from build123d import *

# Parameters (mm, degrees)
F0_W      = 140
F0_H      = 180
F1_DEPTH  = 70
F2_W      = 130
F2_H      = 170
F3_DEPTH  = 65
F4_SIZE   = 45
F5_W      = 30
F5_H      = 49.6265143156
F6_DEPTH  = 25
F7_R      = 14.99999
F9_DEPTH  = 7
F10_W     = 59.1894394159
F10_H     = 26.9657306075
F11_DEPTH = 25
F12_W     = 90
F12_H     = 7
F13_DEPTH = 20
F14_W     = 90
F14_H     = 7
F15_DEPTH = 20
F17_DEPTH = 25
F19_DEPTH = 25
F20_R     = 5


# Not quite as in the source:
# - a fillet or chamfer is up to 0.001 mm smaller than in the source, because OpenCascade refuses the exact size


with BuildPart() as f1:
    # F0 (on Top) → F1 (new body)
    with BuildSketch(Plane.XY):
        with Locations((46.5964969993, 53.7995101511)):
            Rectangle(F0_W, F0_H)
    extrude(amount=F1_DEPTH)

    # F2 (on face) → F3 (cut)
    with BuildSketch(Plane(origin=(0, 0, 0), x_dir=(1, 0, 0), z_dir=(0, 0, -1))):
        with Locations((46.5964969993, -53.7995101511)):
            Rectangle(F2_W, F2_H)
    extrude(amount=-F3_DEPTH, mode=Mode.SUBTRACT)

    # F4
    f4_edges = [f1.edges().sort_by_distance(p)[0] for p in [
        (46.596497, 143.79951, 70),
        (46.596497, 138.79951, 65),
    ]]
    chamfer(f4_edges, length=F4_SIZE)

    # F5 (on face) → F6 (cut)
    with BuildSketch(Plane.XZ.offset(36.2004898489)):
        with Locations((46.5964969993, 24.8132571578)):
            Rectangle(F5_W, F5_H)
    extrude(amount=-F6_DEPTH, mode=Mode.SUBTRACT)

    # F7 (radius 15 in the source; OpenCascade refuses exactly that, so slightly less here)
    f7_edges = [f1.edges().sort_by_distance(p)[0] for p in [
        (61.596497, -33.70049, 49.626514),
        (31.596497, -33.70049, 49.626514),
    ]]
    fillet(f7_edges, radius=F7_R)

    # F8 (on face) → F9 (join)
    with BuildSketch(Plane(origin=(0, 0, 0), x_dir=(1, 0, 0), z_dir=(0, 0, -1))):
        Polygon((-23.4035030007, -28.7995101511), (-23.4035030007, -143.7995101511), (116.5964969993, -143.7995101511), (116.5964969993, -28.7995101511), (111.5964969993, -28.7995101511), (111.5964969993, -138.7995101511), (-18.4035030007, -138.7995101511), (-18.4035030007, -28.7995101511), align=None)
    extrude(amount=F9_DEPTH)

    # F10 (on face) → F11 (cut)
    with BuildSketch(Plane(origin=(0, 143.7995101511, 0), x_dir=(-1, 0, 0), z_dir=(0, 1, 0))):
        with Locations((-46.5964969993, 6.4828653038)):
            Rectangle(F10_W, F10_H)
    extrude(amount=-F11_DEPTH, mode=Mode.SUBTRACT)

    # F12 (on face) → F13 (join)
    with BuildSketch(Plane(origin=(-23.4035030007, 0, 0), x_dir=(0, -1, 0), z_dir=(-1, 0, 0))):
        with Locations((-98.7995101511, -3.5)):
            Rectangle(F12_W, F12_H)
    extrude(amount=F13_DEPTH)

    # F14 (on face) → F15 (join)
    with BuildSketch(Plane.YZ.offset(116.5964969993)):
        with Locations((98.7995101511, -3.5)):
            Rectangle(F14_W, F14_H)
    extrude(amount=F15_DEPTH)

    # F16 (on face) → F17 (cut)
    with BuildSketch(Plane.XY):
        with BuildLine():
            ThreePointArc((-33.4035030007, 135.7995101511), (-34.8177165631, 132.3852965888), (-31.4035030007, 133.7995101511))
            ThreePointArc((-31.4035030007, 133.7995101511), (-31.9892894384, 135.2137237135), (-33.4035030007, 135.7995101511))
        make_face()
        with BuildLine():
            ThreePointArc((-33.4035030007, 61.7995101511), (-31.9892894384, 62.3852965888), (-31.4035030007, 63.7995101511))
            ThreePointArc((-31.4035030007, 63.7995101511), (-34.8177165631, 65.2137237135), (-33.4035030007, 61.7995101511))
        make_face()
    extrude(amount=-F17_DEPTH, mode=Mode.SUBTRACT)

    # F18 (on face) → F19 (cut)
    with BuildSketch(Plane.XY):
        with BuildLine():
            ThreePointArc((126.5964969993, 61.7995101511), (128.0107105616, 62.3852965888), (128.5964969993, 63.7995101511))
            ThreePointArc((128.5964969993, 63.7995101511), (125.1822834369, 65.2137237135), (126.5964969993, 61.7995101511))
        make_face()
        with BuildLine():
            ThreePointArc((126.5964969993, 135.7995101511), (125.1822834369, 132.3852965888), (128.5964969993, 133.7995101511))
            ThreePointArc((128.5964969993, 133.7995101511), (128.0107105616, 135.2137237135), (126.5964969993, 135.7995101511))
        make_face()
    extrude(amount=-F19_DEPTH, mode=Mode.SUBTRACT)

    # F20
    f20_edges = [f1.edges().sort_by_distance(p)[0] for p in [
        (-43.403503, 53.79951, -3.5),
        (-43.403503, 143.79951, -3.5),
        (136.596497, 143.79951, -3.5),
        (136.596497, 53.79951, -3.5),
    ]]
    fillet(f20_edges, radius=F20_R)


solid = f1.part
Can you work these out from the model? Positions are in its coordinate system, mm. A direction names the side the tool comes from. Give positions to 0.01 mm unless a question says otherwise; leave off trailing zeros. Order: outer loops, then holes, each group sorted by start corner. A loop starts at its lowest first (then second) coordinate and runs counter-clockwise, first axis right, second up. Notation, with made-up numbers: M 47.5,3 L 75.5,3 A10 cw 75.5,11 Z; hole C 1,7 d7. An arc over 180 degrees is marked long. Use one line per item in the form item = value. Start each with the question number.
Item 1: If we section it at D-D (z = 45): Write out the boundary of the cut face in (x, y), then the cut area to 3 significant figures.
Item 2: For faces 1 (the flat face through (111.596, 53, 30)), 2 (the flat face through (-33, 99, 0)), 3 (the flat face through (17.002, 141, 6)), 4 (the flat face through (-20, -16, 0)), 5 (the flat face through (124, 53.8, -4)), which set-ups out of +Z, -Z, +X, -X, +Y, -Y let a thin tool reach every point of the face, with its end or its side?
Item 3: If we section it at A-A (x = 108.5): Write out the boundary of the cut face in (y, z).
Item 4: Will these pins go through, and if not, where does the flat tip stop? pin 1 Ø22 at (x, y) = (130, 91.5) entering from +Z; pin 2 Ø12 at (x, z) = (80.5, 37.5) entering from +Y; pin 3 Ø4 at (y, z) = (22.5, 36.5) entering from +X; pin 4 Ø3.5 at (x, y) = (126.6, 63.8) entering from -Z.
Item 5: If I drill on line 1 along Y through (x, z) = (92.5, 2); line 2 along X through (y, z) = (75.5, 30); line 3 along X through (y, z) = (64, -0.5), over which ranges is the centre line in solid material (lowest first)?
Item 6: If we section it at B-B (y = 14.5): Write out the boundary of the cut face in (x, z), then the cut area to 3 significant figures.
Item 7: If we section it at C-C (z = 58): Write out the boundary of the cut face in (x, y), then the cut area to 3 significant figures.
Item 8: We'd pull the mould along X, two halves only. Please class faces 6 (the cylindrical face through (-41.978, 55.303, -3.451)), 7 (the flat face through (114, 28.8, -3)), 8 (the flat face through (47, 141, 19.966)), 9 (the flat face through (76.4, 138.8, 6.7)): +X half, -X half, draft (parallel to the pull), parting line (faces both ways), or undercut.
Outcome:
q1.outline = M -23.4,-36.2 L 35.76,-36.2 L 35.76,-31.2 L -18.4,-31.2 L -18.4,113.8 L 111.6,113.8 L 111.6,-31.2 L 57.43,-31.2 L 57.43,-36.2 L 116.6,-36.2 L 116.6,123.8 L -23.4,123.8 Z
q1.area = 3,440 mm2
q2.face_1 = -Z
q2.face_2 = +Z, -X, +Y, -Y
q2.face_3 = -Z, +Y
q2.face_4 = -Z, +X, -X, -Y
q2.face_5 = +Z, -Z, +X, -Y
q3.outline = M -36.2,0 L -31.2,0 L -31.2,65 L 93.8,65 L 138.8,20 L 138.8,-7 L 143.8,-7 L 143.8,25 L 98.8,70 L -36.2,70 Z
q4.pin_1 = 0
q4.pin_2 = 137.3
q4.pin_3 = 116.6
q4.pin_4 = through
q5.line_1 = -36.2 to -31.2, 138.8 to 143.8
q5.line_2 = -23.4 to -18.4, 111.6 to 116.6
q5.line_3 = -43.4 to -35.39, -31.41 to -18.4, 111.6 to 124.61, 128.59 to 136.6
q6.outline = M -23.4,0 L -18.4,0 L -18.4,65 L 111.6,65 L 111.6,0 L 116.6,0 L 116.6,70 L -23.4,70 Z
q6.area = 1,350 mm2
q7.outline = M -23.4,-36.2 L 116.6,-36.2 L 116.6,110.8 L -23.4,110.8 Z; hole M -18.4,-31.2 L 111.6,-31.2 L 111.6,100.8 L -18.4,100.8 Z
q7.area = 3,420 mm2
q8.face_6 = -X half
q8.face_7 = draft
q8.face_8 = undercut
q8.face_9 = undercut
